Verification items for the finished model (mm, model axes). A direction names the side the tool comes from. Coordinates: 2 decimals unless noted, no trailing zeros. Write each loop counter-clockwise with the first axis right and the second up, starting at its lowest first coordinate (ties: lowest second). Pieces come first, ordered by that corner, then holes. Notation, with made-up numbers: (51.25, -10.5) - (90.25, -10.5) arc R27 cw to (90.25, 17.5) - close; hole circle Ø11 at (60, 13). An arc over 180 degrees is marked (long way). Use CSV: the item, a comma, the result in double quotes. Start each with the question number.
```python
from build123d import *

# Parameters (mm, degrees)
SKETCH1_R                = 7.5
BOSS_EXTRUDE2_DEPTH      = 14
CUT_EXTRUDE1_REACH       = 19.564
SKETCH2_R                = 2
BOSS_EXTRUDE3_START      = -7.279118874
BOSS_EXTRUDE3_DEPTH      = 1.03527618
FILLET1_R                = 10
CIRPATTERN1_COUNT        = 3
FILLET1_OF_CIRPATTERN1_R = 10


with BuildPart() as part:
    # Sketch1 → Boss-Extrude2 (new body)
    with BuildSketch(Plane(origin=(0, 0, 0), x_dir=(1, 0, 0), z_dir=(0, 1, 0))):
        with Locations(Location((0, 0, 0), (0, 0, 270))):
            Circle(SKETCH1_R)
    extrude(amount=BOSS_EXTRUDE2_DEPTH)

    # Sketch2 → Cut-Extrude1 (cut, up to next)
    with BuildSketch(Plane(origin=(0, 14, 0), x_dir=(1, 0, 0), z_dir=(0, 1, 0)), mode=Mode.PRIVATE) as cut_extrude1_sk1:
        with Locations(Location((0, 0, 0), (0, 0, 270))):
            Circle(SKETCH2_R)
    cut_extrude1_tool1 = extrude(cut_extrude1_sk1.sketch, amount=-CUT_EXTRUDE1_REACH, mode=Mode.PRIVATE) & part.part
    add(cut_extrude1_tool1.solids().sort_by_distance((0, 14, 0))[0], mode=Mode.SUBTRACT)

    # Boss-Extrude3: read off the stored shape, not the designer's step
    # Boss-Extrude3 outline → Boss-Extrude3 (add)
    with BuildSketch(Plane(origin=(0, 0, 0), x_dir=(0.9659258262890672, 0.2588190451025251, 0), z_dir=(0.25881904510252507, -0.9659258262890672, 0)).offset(BOSS_EXTRUDE3_START)):
        with BuildLine():
            add(Edge.make_bspline(
                [(-5.688266684, 1.344969698), (-4.547659305, 7.389056985), (1.811733316, 7.498803292)],
                knots=[0.18030465, 0.18030465, 0.18030465, 1.551469461, 1.551469461, 1.551469461], degree=2, weights=[1, 0.771122328, 0.993637519]))
            add(Edge.make_bspline(
                [(1.811733316, 7.498803292), (8.171125936, 7.389056985), (9.311733316, 1.344969698)],
                knots=[1.590123193, 1.590123193, 1.590123193, 2.961288004, 2.961288004, 2.961288004], degree=2, weights=[0.993637519, 0.771122328, 1]))
            Line((9.311733316, 1.344969698), (9.311733316, 54.5))
            Line((9.311733316, 54.5), (-5.688266684, 54.5))
            Line((-5.688266684, 54.5), (-5.688266684, 1.344969698))
        make_face()
    boss_extrude3 = extrude(amount=BOSS_EXTRUDE3_DEPTH)

    # Fillet1
    fillet1_edges = [part.edges().sort_by_distance(p)[0] for p in [
        (7.244443697, 8.941142838, 54.5),
    ]]
    fillet(fillet1_edges, radius=FILLET1_R)

    # CirPattern1: Boss-Extrude3 ×3 about axis
    cirpattern1_axis = Axis((0, 0, 0), (0, 1, 0))
    for i in range(1, CIRPATTERN1_COUNT):
        add(boss_extrude3.rotate(cirpattern1_axis, i * 360 / CIRPATTERN1_COUNT))

    # Fillet1 of CirPattern1
    fillet1_of_cirpattern1_edges = [part.edges().sort_by_distance(p)[0] for p in [
        (43.576162658, 8.941142838, -33.523872278),
        (-50.820606355, 8.941142838, -20.976127722),
    ]]
    fillet(fillet1_of_cirpattern1_edges, radius=FILLET1_OF_CIRPATTERN1_R)


solid = part.part
```
Q1. Tool access check on faces 1 (the cylindrical face through (0.33, 6.902, -7.493)), 2 (the flat face through (-44.8, 5.722, -31.405)). Record the directions out of +Z, -Z, +X, -X, +Y, -Y that give a thin tool (end or side, any length) a straight path to the whole face; none if there is none.
Q2. Cross-section at D-D (x = 18.5). Record the cut outline in (y, z), plus the area to 3 significant figures.
Q3. Release check for a two-part mould opening along X. For faces 3 (the flat face through (-23.21, 8.95, -5.04)), 4 (the flat face through (-5, 6, 54.5)), 5 (the flat face through (15.969, 8.948, -17.582)) record: released by +X, released by -X, zero draft, split by the parting line, or undercut.
Q4. Scan lines: line 1 along X through (y, z) = (4, 0); line 2 along X through (y, z) = (5.5, 0); line 3 along Y through (x, z) = (-25.5, -10). Record each from-to range of solid material in increasing order. Write a range as from..to.
Q5. Cross-section at A-A (z = 0). Record the cut outline in (x, y).
Q6. Gauge pin test, flat ends, axial feed: pin 1 (6 mm diameter, centred on y = 11, z = 14.5, fed in from +X); pin 2 (6 mm diameter, centred on x = 28.5, z = -8, fed in from +Y); pin 3 (5 mm diameter, centred on y = 12.5, z = 8, fed in from +X). Record the tip position at first contact, or that the pin passes through.
Q7. Cross-section at B-B (y = 2). Record the cut outline in (x, z), plus the area to 3 significant figures.
Q8. Cross-section at C-C (z = 12). Record the cut outline in (x, y).
Reply:
1,face 1,"none"
1,face 2,"-Z, -X, +Y, -Y"
2,outline,"(4.56, -2.47) - (8.44, -19.2) - (9.44, -18.89) - (5.56, -2.16) - close"
2,area,"17.9 mm^2"
3,face 3,"released by -X"
3,face 4,"zero draft"
3,face 5,"undercut"
4,line 1,"-7.5..-2, 2..7.5"
4,line 2,"-7.5..-2, 2..14.73"
4,line 3,"7.56..8.63"
5,outline,"(-14.76, 8.44) - (-7.5, 7.47) - (-7.5, 0) - (-2, 0) - (-2, 14) - (-7.5, 14) - (-7.5, 8.54) - (-14.22, 9.44) - close; (2, 0) - (7.5, 0) - (7.5, 5.46) - (14.22, 4.56) - (14.76, 5.56) - (7.5, 6.53) - (7.5, 14) - (2, 14) - close"
6,pin 1,"x = 7.38"
6,pin 2,"y = 6.38"
6,pin 3,"x = 5.1"
7,outline,"circle Ø15 at (0, 0); hole circle Ø4 at (0, 0)"
7,area,"164 mm^2"
8,outline,"(-7.38, 5.56) - (-7.11, 4.56) - (7.38, 8.44) - (7.11, 9.44) - close"
